The model under review builds one solid part; all positions refer to its coordinate system, in mm. A direction names the side the tool comes from. Give positions to 0.01 mm unless a question says otherwise; leave off trailing zeros. Order: outer loops, then holes, each group sorted by start corner. A loop starts at its lowest first (then second) coordinate and runs counter-clockwise, first axis right, second up. Notation, with made-up numbers: (41.5, -35.5) - (87.5, -35.5) arc R22 cw to (87.5, 2.5) - close; hole circle Ø10 at (84.5, 37). An arc over 180 degrees is marked (long way). Use a Markdown table: item, result. Add a question column.
```python
from build123d import *

# Parameters (mm, degrees)
SKETCH_2_W            = 666.5
SKETCH_2_H            = 490
EXTRUDE_1_DEPTH       = 500
SKETCH_3_W            = 45
SKETCH_3_H            = 70
EXTRUDE_2_DEPTH       = 80
CUT_EXTRUDE_1_DEPTH   = 800
EXTRUDE_5_DEPTH       = 500
SKETCH_8_R            = 1.5
EXTRUDE_6_DEPTH       = 300
SKETCH_20_W           = 751.278853788
SKETCH_20_H           = 520
CUT_EXTRUDE_5_DEPTH   = 490
SKETCH_22_R           = 12
CUT_EXTRUDE_7_DEPTH   = 15
SKETCH_23_W           = 120
SKETCH_23_H           = 200
CUT_EXTRUDE_8_DEPTH   = 30
SKETCH_24_W           = 20
SKETCH_24_H           = 10
EXTRUDE_10_DEPTH      = 40
SKETCH_25_W           = 20
SKETCH_25_H           = 15
EXTRUDE_11_DEPTH      = 10
EXTRUDE_12_DEPTH      = 12
EXTRUDE_12_DEPTH_BACK = 30
FILLET_1_R            = 5
SKETCH_27_R           = 12
EXTRUDE_13_DEPTH      = 12
SKETCH_28_R           = 12
EXTRUDE_14_DEPTH      = 5
SKETCH_29_R           = 35
EXTRUDE_15_DEPTH      = 70
EXTRUDE_16_DEPTH      = 33
CUT_EXTRUDE_START     = -15
SKETCH_31_R           = 12
CUT_EXTRUDE_9_DEPTH   = 15
SKETCH_32_W           = 426.5
SKETCH_32_H           = 130
CUT_EXTRUDE_10_DEPTH  = 126
SKETCH_33_R           = 45.31
CUT_EXTRUDE_11_DEPTH  = 44
SKETCH_35_W           = 44
SKETCH_35_H           = 40
EXTRUDE_17_DEPTH      = 50
SKETCH_37_W           = 666.5
SKETCH_37_H           = 10
EXTRUDE_19_DEPTH      = 40
SKETCH_38_W           = 120
SKETCH_38_H           = 10
EXTRUDE_20_DEPTH      = 200


with BuildPart() as part:
    # 草图2 → 凸台-拉伸1 (new body)
    with BuildSketch(Plane(origin=(0, 0, 0), x_dir=(1, 0, 0), z_dir=(0, 1, 0))):
        with Locations((333.25, 255)):
            Rectangle(SKETCH_2_W, SKETCH_2_H)
    extrude(amount=EXTRUDE_1_DEPTH)

    # 草图3 → 凸台-拉伸2 (add)
    with BuildSketch(Plane(origin=(0, 500, 0), x_dir=(1, 0, 0), z_dir=(0, 1, 0))):
        with Locations((52.5, 75)):
            Rectangle(SKETCH_3_W, SKETCH_3_H)
        with Locations((52.5, 245)):
            Rectangle(SKETCH_3_W, SKETCH_3_H)
        with Locations((614, 245)):
            Rectangle(SKETCH_3_W, SKETCH_3_H)
        with Locations((614, 75)):
            Rectangle(SKETCH_3_W, SKETCH_3_H)
    extrude(amount=EXTRUDE_2_DEPTH)

    # 草图4 → 切除-拉伸1 (cut)
    with BuildSketch(Plane.ZY.offset(-30)):
        with BuildLine():
            Line((-280, 500), (-264.445556098, 564.676574391))
            ThreePointArc((-264.445556098, 564.676574391), (-245, 580), (-225.554443902, 564.676574391))
            Line((-225.554443902, 564.676574391), (-210, 500))
            Line((-210, 500), (-110, 500))
            Line((-110, 500), (-94.445556098, 564.676574391))
            ThreePointArc((-94.445556098, 564.676574391), (-75, 580), (-55.554443902, 564.676574391))
            Line((-55.554443902, 564.676574391), (-40, 500))
            Line((-40, 500), (-40, 590.908516605))
            Line((-40, 590.908516605), (-280, 590.908516605))
            Line((-280, 590.908516605), (-280, 580))
            Line((-280, 580), (-280, 500))
        make_face()
    extrude(amount=-CUT_EXTRUDE_1_DEPTH, mode=Mode.SUBTRACT)

    # 草图7 → 凸台-拉伸5 (add)
    with BuildSketch(Plane(origin=(0, 500, 0), x_dir=(1, 0, 0), z_dir=(0, 1, 0))):
        Polygon((476.5, 370), (546.5, 370), (546.5, 350), (476.5, 350), (120, 350), (120, 370), align=None)
    extrude(amount=EXTRUDE_5_DEPTH)

    # 草图8 → 凸台-拉伸6 (add)
    with BuildSketch(Plane.XY.offset(-350)):
        with Locations(Location((155, 832, 0), (0, 0, 180))):
            Circle(SKETCH_8_R)
        with Locations(Location((511.5, 832, 0), (0, 0, 180))):
            Circle(SKETCH_8_R)
        Polygon((177, 805), (177, 813), (166, 813), (166, 819), (170, 819), (170, 827), (140, 827), (140, 819), (144, 819), (144, 813), (133, 813), (133, 805), align=None)
        Polygon((500.5, 813), (489.5, 813), (489.5, 805), (533.5, 805), (533.5, 813), (522.5, 813), (522.5, 819), (526.5, 819), (526.5, 827), (496.5, 827), (496.5, 819), (500.5, 819), align=None)
    extrude(amount=EXTRUDE_6_DEPTH)

    # 草图20 → 切除-拉伸5 (cut)
    with BuildSketch(Plane.XZ):
        with Locations((375.639426894, -260)):
            Rectangle(SKETCH_20_W, SKETCH_20_H)
    extrude(amount=-CUT_EXTRUDE_5_DEPTH, mode=Mode.SUBTRACT)

    # 草图22 → 切除-拉伸7 (cut)
    # profile 1 of 2: a face of its own
    with BuildSketch(Plane.ZY.offset(-45)):
        with BuildLine():
            Line((-264.44592578, 564.676479403), (-273.266117859, 528))
            Line((-273.266117859, 528), (-216.733882141, 528))
            Line((-216.733882141, 528), (-225.52728646, 564.563651658))
            ThreePointArc((-225.52728646, 564.563651658), (-244.942017925, 580.000253177), (-264.44592578, 564.676479403))
        make_face()
        with Locations((-245, 560)):
            Circle(SKETCH_22_R, mode=Mode.SUBTRACT)
    # profile 2 of 2: a face of its own
    with BuildSketch(Plane.ZY.offset(-45)):
        with BuildLine():
            ThreePointArc((-55.55407422, 564.676479403), (-75.057982075, 580.000253177), (-94.47271354, 564.563651658))
            Line((-94.47271354, 564.563651658), (-103.266117859, 528))
            Line((-103.266117859, 528), (-46.733882141, 528))
            Line((-46.733882141, 528), (-55.55407422, 564.676479403))
        make_face()
        with Locations((-75, 560)):
            Circle(SKETCH_22_R, mode=Mode.SUBTRACT)
    extrude(amount=-CUT_EXTRUDE_7_DEPTH, mode=Mode.SUBTRACT)

    # 草图23 → 切除-拉伸8 (cut)
    with BuildSketch(Plane(origin=(0, 500, 0), x_dir=(1, 0, 0), z_dir=(0, 1, 0))):
        with Locations((606.5, 400)):
            Rectangle(SKETCH_23_W, SKETCH_23_H)
        with Locations((60, 400)):
            Rectangle(SKETCH_23_W, SKETCH_23_H)
    extrude(amount=-CUT_EXTRUDE_8_DEPTH, mode=Mode.SUBTRACT)

    # 草图24 → 凸台-拉伸10 (add)
    with BuildSketch(Plane.XY.offset(-350)):
        with Locations((210, 945)):
            Rectangle(SKETCH_24_W, SKETCH_24_H)
    extrude(amount=EXTRUDE_10_DEPTH)

    # 草图25 → 凸台-拉伸11 (add)
    with BuildSketch(Plane(origin=(0, 950, 0), x_dir=(1, 0, 0), z_dir=(0, 1, 0))):
        with Locations((210, 317.5)):
            Rectangle(SKETCH_25_W, SKETCH_25_H)
    extrude(amount=EXTRUDE_11_DEPTH)

    # 草图26 → 凸台-拉伸12 (add, two sides: drawn at the far end of the back side and taken through both)
    with BuildSketch(Plane(origin=(0, 141.807806183, -529.233937587), x_dir=(1, 0, 0), z_dir=(0, -0.25881904510252135, 0.9659258262890681)).offset(-EXTRUDE_12_DEPTH_BACK)):
        Polygon((190, 839.594999439), (190, 869.594999439), (230, 869.594999439), (230, 839.594999439), (230, 835.594999439), (190, 835.594999439), align=None)
    extrude(amount=EXTRUDE_12_DEPTH + EXTRUDE_12_DEPTH_BACK)

    # 圆角1
    fillet_1_edges = [part.edges().sort_by_distance(p)[0] for p in [
        (230, 951.259967865, -321.659370176),
        (190, 951.259967865, -321.659370176),
        (190, 984.101445959, -312.859522643),
        (230, 984.101445959, -312.859522643),
    ]]
    fillet(fillet_1_edges, radius=FILLET_1_R)

    # 草图27 → 凸台-拉伸13 (add)
    with BuildSketch(Plane(origin=(0, 138.701977642, -517.642827671), x_dir=(1, 0, 0), z_dir=(0, -0.25881904510252535, 0.9659258262890672))):
        with Locations(Location((210, 852.594999439, 0), (0, 0, 270))):
            Circle(SKETCH_27_R)
    extrude(amount=EXTRUDE_13_DEPTH)

    # 草图28 → 凸台-拉伸14 (add)
    with BuildSketch(Plane(origin=(75, 0, 0), x_dir=(0, 0, -1), z_dir=(1, 0, 0))):
        with Locations(Location((245, 560, 0), (0, 0, 180))):
            Circle(SKETCH_28_R)
    extrude(amount=EXTRUDE_14_DEPTH)

    # 草图29 → 凸台-拉伸15 (add)
    with BuildSketch(Plane(origin=(80, 0, 0), x_dir=(0, 0, -1), z_dir=(1, 0, 0))):
        with Locations((245, 560)):
            Circle(SKETCH_29_R)
    extrude(amount=EXTRUDE_15_DEPTH)

    # 草图30 → 凸台-拉伸16 (add)
    with BuildSketch(Plane(origin=(0, 500, 0), x_dir=(1, 0, 0), z_dir=(0, 1, 0))):
        Polygon((128, 265), (138, 265), (138, 225), (128, 225), (88, 225), (88, 233), (88, 257), (88, 265), align=None)
    extrude(amount=EXTRUDE_16_DEPTH)

    # 草图31 → 切除-拉伸9 (cut)
    # profile 1 of 2: a face of its own
    with BuildSketch(Plane(origin=(621.5, 0, 0), x_dir=(0, 0, -1), z_dir=(1, 0, 0)).offset(CUT_EXTRUDE_START)):
        with BuildLine():
            Line((55.55407422, 564.676479403), (46.733882141, 528))
            Line((46.733882141, 528), (103.266117859, 528))
            Line((103.266117859, 528), (94.47271354, 564.563651658))
            ThreePointArc((94.47271354, 564.563651658), (75.057982075, 580.000253177), (55.55407422, 564.676479403))
        make_face()
        with Locations(Location((75, 560, 0), (0, 0, 180))):
            Circle(SKETCH_31_R, mode=Mode.SUBTRACT)
    # profile 2 of 2: a face of its own
    with BuildSketch(Plane(origin=(621.5, 0, 0), x_dir=(0, 0, -1), z_dir=(1, 0, 0)).offset(CUT_EXTRUDE_START)):
        with BuildLine():
            ThreePointArc((264.44592578, 564.676479403), (244.942017925, 580.000253177), (225.52728646, 564.563651658))
            Line((225.52728646, 564.563651658), (216.733882141, 528))
            Line((216.733882141, 528), (273.266117859, 528))
            Line((273.266117859, 528), (264.44592578, 564.676479403))
        make_face()
        with Locations(Location((245, 560, 0), (0, 0, 180))):
            Circle(SKETCH_31_R, mode=Mode.SUBTRACT)
    extrude(amount=CUT_EXTRUDE_9_DEPTH, mode=Mode.SUBTRACT)

    # 草图32 → 切除-拉伸10 (cut)
    with BuildSketch(Plane(origin=(0, 500, 0), x_dir=(1, 0, 0), z_dir=(0, 1, 0))):
        with Locations((333.25, 435)):
            Rectangle(SKETCH_32_W, SKETCH_32_H)
    extrude(amount=-CUT_EXTRUDE_10_DEPTH, mode=Mode.SUBTRACT)

    # 草图33 → 切除-拉伸11 (cut, along a direction that is not the sketch's normal)
    with BuildSketch(Plane.XY.offset(-350)):
        with Locations((462, 926.518617387)):
            Circle(SKETCH_33_R)
    extrude(amount=-CUT_EXTRUDE_11_DEPTH, dir=(5.875812413124604e-15, -0.031880547720424424, 0.9994916861470363), mode=Mode.SUBTRACT)

    # 草图35 → 凸台-拉伸17 (add)
    with BuildSketch(Plane.XY.offset(-50)):
        with Locations((155, 825)):
            Rectangle(SKETCH_35_W, SKETCH_35_H)
        with Locations((511.5, 825)):
            Rectangle(SKETCH_35_W, SKETCH_35_H)
    extrude(amount=EXTRUDE_17_DEPTH)

    # 草图37 → 凸台-拉伸19 (add)
    with BuildSketch(Plane.XY.offset(-10)):
        with Locations((333.25, 495)):
            Rectangle(SKETCH_37_W, SKETCH_37_H)
    extrude(amount=EXTRUDE_19_DEPTH)

    # 草图38 → 凸台-拉伸20 (add)
    with BuildSketch(Plane(origin=(0, 0, -300), x_dir=(-1, 0, 0), z_dir=(0, 0, -1))):
        with Locations((-606.5, 495)):
            Rectangle(SKETCH_38_W, SKETCH_38_H)
        with Locations((-60, 495)):
            Rectangle(SKETCH_38_W, SKETCH_38_H)
    extrude(amount=EXTRUDE_20_DEPTH)


solid = part.part
```
Q1. We need section B-B (z = -245). Count the separate pieces of the cut face and the enclosed holes in it, plus the area to 3 significant figures.
Q2. Wall thickness on probe 1 along Y at (x, z) = (500, -147); probe 2 along Y at (x, z) = (41.5, -157.5); probe 3 along Z at (x, y) = (179.5, 682.5): over which ranges is each line inside the solid? List them lowest first.
Q3. We need section C-C (x = 257). Write out the cut boundary in (y, z), plus the area to 3 significant figures.
Q4. We need section A-A (z = -398). Write out the cut boundary in (x, y).
Q5. Machinability: for faces 4 (the flat face through (613.68, 524.7, -104.06)), 5 (the flat face through (621.5, 543, -75)), 6 (the flat face through (511, 825, 0)), which of the approach directions +Z, -Z, +X, -X, +Y, -Y give a long, thin tool a straight path to every point of the face, cutting with its end or side? Answer none if there is none.
Q6. Draft analysis for pull direction X (two halves, no side actions). For faces 1 (the flat face through (621.5, 543, -245)), 2 (the flat face through (190, 968, -317)), 3 (the flat face through (230, 968, -318)), state which applies: pulls with the +X half, pulls with the -X half, needs draft (parallel to the pull), parting line crosses it, or undercut.
Q7. Clearance check with flat-ended pins moving along their axes: P1, Ø6.5, axis at y = 815, z = -184, coming from the +X side; P2, Ø12, axis at x = 165, y = 786.5, coming from the +Z side; P3, Ø4, axis at x = 447.5, y = 862, coming from the -Z side. State where each tip first meets the part, or that it passes through.
Q8. We need section D-D (y = 620.5). Write out the cut boundary in (x, z), plus the area to 3 significant figures.
Here are the results:
| question | item | result |
|---|---|---|
| 1 | separate pieces | 5 |
| 1 | enclosed holes | 3 |
| 1 | area | 20,800 mm2 |
| 2 | probe 1 | 490 to 500, 805 to 813, 819 to 827 |
| 2 | probe 2 | 490 to 500 |
| 2 | probe 3 | -370 to -350 |
| 3 | outline | (490, -370) - (1000, -370) - (1000, -350) - (500, -350) - (500, 30) - (490, 30) - close |
| 3 | area | 14,000 mm2 |
| 4 | outline | (0, 490) - (120, 490) - (120, 500) - (0, 500) - close; (546.5, 490) - (666.5, 490) - (666.5, 500) - (546.5, 500) - close |
| 5 | face 4 | +X, -X, +Y |
| 5 | face 5 | none |
| 5 | face 6 | +Z, +X, -X, +Y |
| 6 | face 1 | undercut |
| 6 | face 2 | pulls with the -X half |
| 6 | face 3 | pulls with the +X half |
| 7 | P1 | x = 533.5 |
| 7 | P2 | z = -350 |
| 7 | P3 | z = -370 |
| 8 | outline | (120, -370) - (546.5, -370) - (546.5, -350) - (120, -350) - close |
| 8 | area | 8,530 mm2 |
